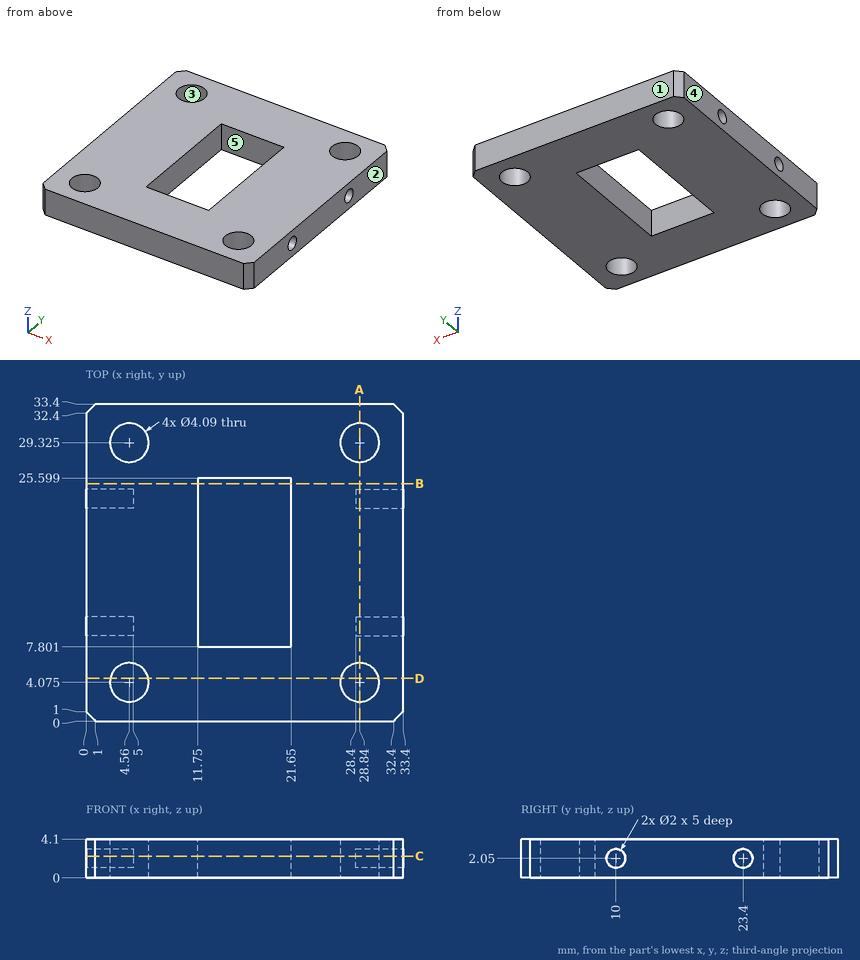
Answer from the drawing. Dimensions are ordinates in mm from the lowest x, y and z of the part. A direction names the side the tool comes from. Coordinates: 2 decimals unless noted, no trailing zeros. Order: outer loops, then holes, each group sorted by start corner. A loop starts at its lowest first (then second) coordinate and runs counter-clockwise, first axis right, second up. Notation, with made-up numbers: (12.25, -26.5) - (65.25, -26.5) arc R21 cw to (65.25, -16.5) - close; hole circle Ø5 at (-16, 88.5). An arc over 180 degrees is marked (long way). Answer as a JSON object with one key per item and string values. Group by question number.
Item 1: Section C-C (z = 2.3) is taken. State how many separate pieces and enclosed holes the cut face has, plus the area to 3 significant figures.
Item 2: Section B-B (y = 25) is taken. Give the vertices of the cut face in (x, z).
Item 3: Consider probe 1 along Y at (x, z) = (1.6, 2.05); probe 2 along Y at (x, z) = (28.84, 2); probe 3 along Y at (x, z) = (18, 1.35). Determine where each line is inside the solid, lowest interval first. Write a range as from..to.
Item 4: Section A-A (x = 28.84) is taken. Give the vertices of the cut face in (y, z).
Item 5: The mould has two halves that part along Y. Classify the marked faces 1, 2 and 3: +Y half, -Y half, draft (parallel to the pull), parting line (faces both ways), or undercut.
Item 6: A tool of negligible diameter and unlimited length cuts with its end or side. For the marked faces 4 and 5, from which of +Z, -Z, +X, -X, +Y, -Y can it reach the whole face along a straight path? Write none if from no direction.
Item 7: Section D-D (y = 4.5) is taken. Give the vertices of the cut face in (x, z), plus the area to 3 significant figures.
Item 8: Flat-ended cylindrical pins translate along their axes: P1, Ø2, axis at x = 14.5, z = 2.5, coming from the -Y side; P2, Ø0.6, axis at y = 10, z = 2.5, coming from the +X side; P3, Ø0.6, axis at y = 10, z = 2.5, coming from the -X side. Find the tip coordinate at first contact, or state that the pin passes through.
Results are:
{
 "1": {"separate pieces": "1", "enclosed holes": "5", "area": "846 mm^2"},
 "2": {"outline": "(0, 0) - (11.75, 0) - (11.75, 4.1) - (0, 4.1) - close; (21.65, 0) - (33.4, 0) - (33.4, 4.1) - (21.65, 4.1) - close"},
 "3": {"probe 1": "y = 0..9, 11..22.4, 24.4..33.4", "probe 2": "y = 0..2.03, 6.12..9, 11..22.4, 24.4..27.28, 31.37..33.4", "probe 3": "y = 0..7.8, 25.6..33.4"},
 "4": {"outline": "(0, 0) - (2.03, 0) - (2.03, 4.1) - (0, 4.1) - close; (6.12, 0) - (27.28, 0) - (27.28, 4.1) - (6.12, 4.1) - close; (31.37, 0) - (33.4, 0) - (33.4, 4.1) - (31.37, 4.1) - close; hole circle Ø2 at (10, 2.05); hole circle Ø2 at (23.4, 2.05)"},
 "5": {"face 1": "+Y half", "face 2": "draft", "face 3": "undercut"},
 "6": {"face 4": "+Z, -Z, -X, +Y, -Y", "face 5": "+Z, -Z"},
 "7": {"outline": "(0, 0) - (2.56, 0) - (2.56, 4.1) - (0, 4.1) - close; (6.56, 0) - (26.84, 0) - (26.84, 4.1) - (6.56, 4.1) - close; (30.84, 0) - (33.4, 0) - (33.4, 4.1) - (30.84, 4.1) - close", "area": "104 mm^2"},
 "8": {"P1": "stops at y = 0", "P2": "stops at x = 28.4", "P3": "stops at x = 5"}
}
